Input: part model. Units: mm. Frame: model coordinates. Face numbers are marked on the shaded views. A direction names the side the tool comes from. Coordinates: 2 decimals unless noted, no trailing zeros. Order: outer loops, then holes, each group sorted by start corner. A loop starts at its lowest first (then second) coordinate and runs counter-clockwise, first axis right, second up. Notation, with made-up numbers: M 56,86 L 91,86 A27 ccw 91,114 Z; hole C -38.75,68.5 d10. An arc over 180 degrees is marked long. One line per item, written item: value.
```python
from build123d import *

# Parameters (mm, degrees)
F2_W     = 56
F2_H     = 56
F3_DEPTH = 2
F2_W_2   = 60
F2_H_2   = 60
F4_DEPTH = 70
F5_R     = 5
F6_R     = 3


with BuildPart() as f3:
    # F2 (on Top) → F3 (new body)
    with BuildSketch(Plane.XY):
        Rectangle(F2_W, F2_H)
    extrude(amount=F3_DEPTH)

    # F2 (on Top) → F4 (join)
    with BuildSketch(Plane.XY):
        Rectangle(F2_W_2, F2_H_2)
        Rectangle(F2_W, F2_H, mode=Mode.SUBTRACT)
    extrude(amount=F4_DEPTH)

    # F5
    f5_edges = [f3.edges().sort_by_distance(p)[0] for p in [
        (30, -30, 35),
        (-30, -30, 35),
        (30, 30, 35),
        (-30, 30, 35),
    ]]
    fillet(f5_edges, radius=F5_R)

    # F6
    f6_edges = [f3.edges().sort_by_distance(p)[0] for p in [
        (-28, 28, 36),
        (28, 28, 36),
        (28, -28, 36),
        (-28, -28, 36),
    ]]
    fillet(f6_edges, radius=F6_R)


solid = f3.part
```
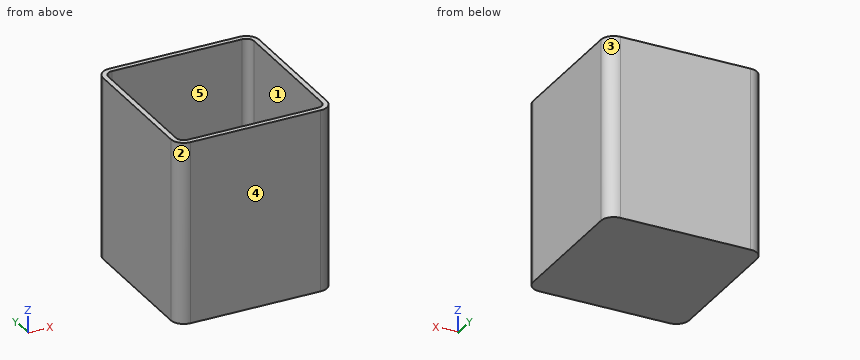
(1) Access query for the marked faces 4 and 5. Directions: +Z, -Z, +X, -X, +Y, -Y. A direction counts if a zero-diameter tool reaches every point of the face in a straight line with its end or side. Return the directions, or none.
Data:
face 4: +Z, -Z, +X, -X, -Y
face 5: +Z
(2) Cut plane B-B on x = -19. Output: boundary loops of the cut face in (y, z), plus the area to 3 significant figures.
Data:
outline: M -30,0 L 30,0 L 30,70 L 28,70 L 28,2 L -28,2 L -28,70 L -30,70 Z
area: 392 mm2
(3) Cut plane A-A on z = 54. Output: boundary loops of the cut face in (x, y), plus the area to 3 significant figures.
Data:
outline: M -30,-25 A5 ccw -25,-30 L 25,-30 A5 ccw 30,-25 L 30,25 A5 ccw 25,30 L -25,30 A5 ccw -30,25 Z; hole M -28,-25 A3 ccw -25,-28 L 25,-28 A3 ccw 28,-25 L 28,25 A3 ccw 25,28 L -25,28 A3 ccw -28,25 Z
area: 450 mm2
(4) Ray query, line 1 (X direction, y = -21, z = 13.5); line 2 (Y direction, x = -26, z = 40.5). Return the intervals inside material, ascending. Write a range as from..to.
Data:
line 1: x = -30..-28, 28..30
line 2: y = -29.9..-27.83, 27.83..29.9
(5) First-contact query: pin 1 (1.5 mm diameter, centred on x = 22.5, y = -5.5, fed in from +Z). Flat tip, straight axial feed; report the tip coordinate or a pass-through.
Data:
pin 1: stops at z = 2
(6) Draft query along X for the marked faces 1, 2 and 3. Return one class per face: released by +X, released by -X, zero draft, split by the parting line, or undercut.
Data:
face 1: undercut
face 2: released by -X
face 3: released by +X
